from build123d import *

# Parameters (mm, degrees)
F1_DEPTH = 12.7
F2_R     = 4.0005
F3_DEPTH = 12.7


with BuildPart() as f1:
    # F0 (on Front) → F1 (new body)
    with BuildSketch(Plane.XZ):
        with BuildLine():
            ThreePointArc((3.989522, 0.864604), (1.185338, -0.11271), (-1.782134, 0))
            Line((-1.782134, 0), (-29.999, 0))
            ThreePointArc((-29.999, 0), (-32.342439, -5.657561), (-38, -8.001))
            Line((-38, -8.001), (-11.422469, -8.001))
            Line((-11.422469, -8.001), (3.989522, 0.864604))
        make_face()
        with BuildLine():
            Line((-29.999, 0), (-1.782134, 0))
            ThreePointArc((-1.782134, 0), (-7.965707, 7.049325), (-3.207935, 15.129744))
            Line((-3.207935, 15.129744), (-19.496256, 8.001))
            Line((-19.496256, 8.001), (-38, 8.001))
            ThreePointArc((-38, 8.001), (-32.342439, 5.657561), (-29.999, 0))
        make_face()
        with BuildLine():
            ThreePointArc((-3.207935, 15.129744), (-7.965707, 7.049325), (-1.782134, 0))
            ThreePointArc((-1.782134, 0), (1.185338, -0.11271), (3.989522, 0.864604))
            ThreePointArc((3.989522, 0.864604), (6.925899, 3.794015), (8.001, 7.8))
            ThreePointArc((8.001, 7.8), (4.378888, 14.496368), (-3.207935, 15.129744))
        make_face()
        with BuildLine():
            ThreePointArc((-38, -8.001), (-32.342439, -5.657561), (-29.999, 0))
            ThreePointArc((-29.999, 0), (-32.342439, 5.657561), (-38, 8.001))
            ThreePointArc((-38, 8.001), (-46.001, 0), (-38, -8.001))
        make_face()
    extrude(amount=F1_DEPTH)

    # F2 (on face) → F3 (cut, through all)
    with BuildSketch(Plane.XZ.offset(12.7)):
        with Locations((-38, 0)):
            Circle(F2_R)
        with Locations((0, 7.8)):
            Circle(F2_R)
    extrude(amount=-F3_DEPTH, mode=Mode.SUBTRACT)


solid = f1.part
CAD build for the part. Positions are in the model's coordinates, mm. A direction names the side the tool comes from. Give positions to 0.01 mm unless a question says otherwise; leave off trailing zeros. Write each loop counter-clockwise with the first axis right and the second up, starting at its lowest first coordinate (ties: lowest second). Pieces come first, ordered by that corner, then holes. Notation, with made-up numbers: M 9.25,13.5 L 14.25,13.5 A19 cw 14.25,32.5 Z; hole C 1,26 d4. An arc over 180 degrees is marked long. Put each result on its own line as item: value. Start each with the question number.
(1) Band-saw the part on C-C, the plane z = 10.75. Write the cut outline in (x, y), and give its area (3 significant figures).
(2) Flat gauge pins, fed straight in: pin 1 Ø1.5 at (y, z) = (-4, -5.5) entering from -X; pin 2 Ø3 at (y, z) = (-10.5, -2) entering from -X. Where does each tip first touch, or does it go through?
(3) Mould opens along X. For faces 1 (the face through (2.151, -6.439, 11.173)), 2 (the face through (-19, 0, 1)), 3 (the face through (-46, -6, 0)) say: +X half, -X half, draft (parallel to the pull), parting line (faces both ways), or undercut.
(4) Band-saw the part on B-B, the plane x = 0. Write the cut outline in (y, z).
(5) Band-saw the part on D-D, the plane x = -20.5. Write the cut outline in (y, z).
(6) Which spindle directions (+Z, -Z, +X, -X, +Y, -Y) get a long thin tool onto all of the face, cutting with end or side? Do faces 4 (the face through (-42, -6, 0)), 5 (the face through (-29, -6, 8.001)). Say none if no direction does.
(7) Probe L1, parallel to Z at x = -38, y = -8.25; L2, parallel to Z at x = -2, y = -6.25; L3, parallel to Z at x = -24, y = -11.25. List the from-to ranges inside material, lowest first.
(8) Band-saw the part on A-A, the plane y = -4.75. Write the cut outline in (x, z).
Response values:
1. outline: M -13.22,-12.7 L -2.7,-12.7 L -2.7,0 L -13.22,0 Z; M 2.7,-12.7 L 7.44,-12.7 L 7.44,0 L 2.7,0 Z
1. area: 194 mm2
2. pin 1: stops at x = -44.44
2. pin 2: stops at x = -45.99
3. face 1: undercut
3. face 2: draft
3. face 3: -X half
4. outline: M -12.7,-1.43 L 0,-1.43 L 0,3.8 L -12.7,3.8 Z; M -12.7,11.8 L 0,11.8 L 0,15.8 L -12.7,15.8 Z
5. outline: M -12.7,-8 L 0,-8 L 0,8 L -12.7,8 Z
6. face 4: +Y, -Y
6. face 5: +Z, -X, +Y, -Y
7. L1: z = -8 to -4, 4 to 8
7. L2: z = -2.58 to 4.34, 11.26 to 15.55
7. L3: z = -8 to 8
8. outline: M -38,-8 L -11.42,-8 L 3.99,0.86 A8 ccw 8,7.8 A8 ccw -3.21,15.13 L -19.5,8 L -38,8 A8 ccw Z; hole C -38,0 d8; hole C 0,7.8 d8
